Build history of the part. All positions in model axes, mm. A direction names the side the tool comes from. Give positions to 0.01 mm unless a question says otherwise; leave off trailing zeros. Write each loop counter-clockwise with the first axis right and the second up, starting at its lowest first coordinate (ties: lowest second). Pieces come first, ordered by that corner, then holes. Notation, with made-up numbers: M 16.5,-25.5 L 56.5,-25.5 A28 ccw 56.5,-6.5 Z; hole C 18,-10.75 d6. An arc over 180 degrees is marked long. One line per item, written item: value. Start each with the question number.
from build123d import *

# Parameters (mm, degrees)
SKETCH1_W                = 29
SKETCH1_H                = 29
BOSS_EXTRUDE1_DEPTH      = 2
SKETCH2_W                = 29
SKETCH2_H                = 2
BOSS_EXTRUDE2_DEPTH      = 27
SKETCH4_R                = 2.5
CUT_EXTRUDE1_DEPTH       = 30
SKETCH6_R                = 2.5
BOSS_EXTRUDE3_DEPTH      = 1
BOSS_EXTRUDE3_DEPTH_BACK = 1


with BuildPart() as part:
    # Sketch1 → Boss-Extrude1 (new body)
    with BuildSketch(Plane(origin=(0, 0, 0), x_dir=(1, 0, 0), z_dir=(0, 1, 0))):
        Rectangle(SKETCH1_W, SKETCH1_H)
    extrude(amount=BOSS_EXTRUDE1_DEPTH)

    # Sketch2 → Boss-Extrude2 (add)
    with BuildSketch(Plane(origin=(0, 2, 0), x_dir=(1, 0, 0), z_dir=(0, 1, 0))):
        with Locations((0, -13.5)):
            Rectangle(SKETCH2_W, SKETCH2_H)
    boss_extrude2 = extrude(amount=BOSS_EXTRUDE2_DEPTH)

    # Mirror1: Boss-Extrude2 across plane
    add(boss_extrude2.mirror(Plane.XY))

    # Sketch4 → Cut-Extrude1 (cut, through all)
    with BuildSketch(Plane.XY.offset(14.5)):
        with Locations((0, 15.5)):
            Circle(SKETCH4_R)
    extrude(amount=-CUT_EXTRUDE1_DEPTH, mode=Mode.SUBTRACT)

    # Sketch6 → Boss-Extrude3 (add, two sides)
    with BuildSketch(Plane(origin=(0, 0, 0), x_dir=(0, 0, -1), z_dir=(1, 0, 0))) as boss_extrude3_sk:
        with BuildLine():
            Line((-12.340534921, 0), (12.662436349, 0))
            Line((12.662436349, 0), (4.632980363, -16.057003584))
            ThreePointArc((4.632980363, -16.057003584), (0.160950714, -18.820723008), (-4.311078935, -16.057003584))
            Line((-4.311078935, -16.057003584), (-12.340534921, 0))
        make_face()
        with Locations((0.160950714, -13.820723008)):
            Circle(SKETCH6_R, mode=Mode.SUBTRACT)
    extrude(amount=BOSS_EXTRUDE3_DEPTH)
    extrude(boss_extrude3_sk.sketch, amount=-BOSS_EXTRUDE3_DEPTH_BACK)


solid = part.part
1) Band-saw the part on C-C (y = 23.5). List the corners of the cut face in (x, z), then the cut area to 3 significant figures.
2) Band-saw the part on B-B (x = 0). List the corners of the cut face in (y, z).
3) Mould opens along X. For faces 1 (the face through (-0.54, 13.06, -13.49)), 2 (the face through (14.5, 1.5, -2.2)), 3 (the face through (-0.01, -16.26, 0.38)), 4 (the face through (-14.5, 1.5, -2.2)) say: released by +X, released by -X, zero draft, split by the parting line, or undercut.
4) Band-saw the part on D-D (z = -0.75). List the corners of the cut face in (x, y), then the cut area to 3 significant figures.
5) Probe line 1 along Z through (x, y) = (-6.5, 24); line 2 along Y through (x, z) = (0, 13.15); line 3 along Y through (x, z) = (-12.25, 8). List the from-to ranges inside material, lowest first. Write a range as from..to.
6) Band-saw the part on A-A (y = 17). List the corners of the cut face in (x, z), then the cut area to 3 significant figures.
7) Drop flat-ended pins along their axis: P1, Ø4, axis at x = -11.5, z = 0.5, coming from the +Y side; P2, Ø15, axis at y = -8.5, z = -3.5, coming from the -X side; P3, Ø15, axis at y = -13, z = 1.5, coming from the +X side. Give the stop position or say it passes through.
8) Tool access for faces 5 (the face through (-1, -7, 0)), 6 (the face through (0.01, -7.92, -8.7)), 7 (the face through (0, 2, 0)), 8 (the face through (1, -7, 0)): list every direction of +Z, -Z, +X, -X, +Y, -Y with a clear straight run to the whole face (end or side of a thin tool).
Model answer:
1. outline: M -14.5,-14.5 L 14.5,-14.5 L 14.5,-12.5 L -14.5,-12.5 Z; M -14.5,12.5 L 14.5,12.5 L 14.5,14.5 L -14.5,14.5 Z
1. area: 116 mm²
2. outline: M -16.06,-4.63 L 0,-12.66 L 0,-14.5 L 13,-14.5 L 13,-12.5 L 2,-12.5 L 2,12.5 L 13,12.5 L 13,14.5 L 0,14.5 L 0,12.34 L -16.06,4.31 A5 ccw Z; M 18,-14.5 L 29,-14.5 L 29,-12.5 L 18,-12.5 Z; M 18,12.5 L 29,12.5 L 29,14.5 L 18,14.5 Z; hole C -13.82,-0.16 d5
3. face 1: undercut
3. face 2: released by +X
3. face 3: zero draft
3. face 4: released by -X
4. outline: M -14.5,0 L -1,0 L -1,-11.39 L 1,-11.39 L 1,0 L 14.5,0 L 14.5,2 L -14.5,2 Z; M -1,-18.79 L 1,-18.79 L 1,-16.25 L -1,-16.25 Z
4. area: 85.9 mm²
5. line 1: z = -14.5..-12.5, 12.5..14.5
5. line 2: y = 0..13, 18..29
5. line 3: y = 0..2
6. outline: M -14.5,-14.5 L -2,-14.5 L -2,-12.5 L -14.5,-12.5 Z; M -14.5,12.5 L -2,12.5 L -2,14.5 L -14.5,14.5 Z; M 2,-14.5 L 14.5,-14.5 L 14.5,-12.5 L 2,-12.5 Z; M 2,12.5 L 14.5,12.5 L 14.5,14.5 L 2,14.5 Z
6. area: 100 mm²
7. P1: stops at y = 2
7. P2: stops at x = -1
7. P3: stops at x = 1
8. face 5: +Z, -Z, -X, -Y
8. face 6: -Z, +X, -X, -Y
8. face 7: +X, -X, +Y
8. face 8: +Z, -Z, +X, -Y
